Geometry: see drawing. Coordinates: mm, zero at the bounding-box minimum. A direction names the side the tool comes from. Coordinates: 2 decimals unless noted, no trailing zeros. Loops run counter-clockwise (first coordinate to the right, second up) from the corner with the lowest first, then second, coordinate; pieces in that order, holes last. Notation, with made-up numbers: (7.25, 13.25) - (57.25, 13.25) arc R17 ccw to (57.25, 35.25) - close; hole circle Ø8 at (-30.75, 9.25). An arc over 180 degrees is marked (long way). Answer in a Markdown table with one row per item.
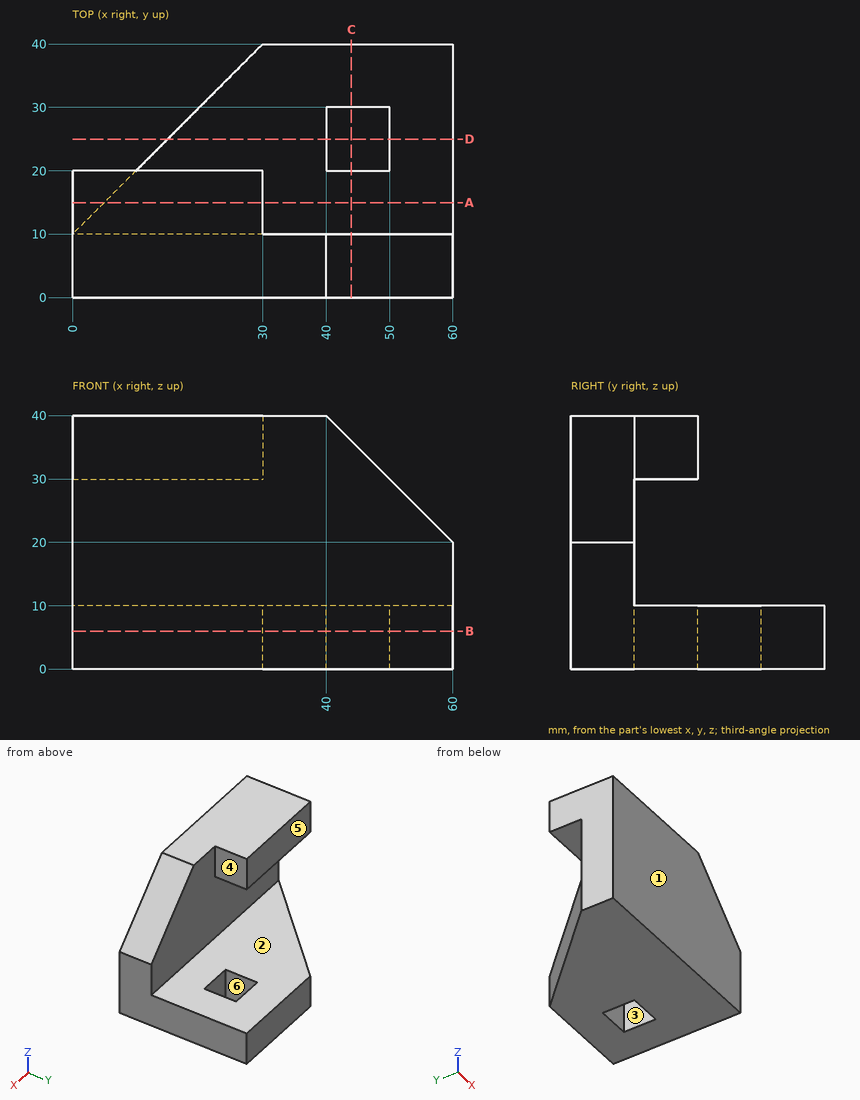
(1) Pull-direction query (Y, two-part tool) for the marked faces 4, 5 and 6; classes: pulls with the +Y half, pulls with the -Y half, needs draft (parallel to the pull), parting line crosses it, or undercut.
Verdict:
| item | result |
|---|---|
| face 4 | needs draft |
| face 5 | pulls with the +Y half |
| face 6 | undercut |
(2) Cut plane C-C on x = 44. Output: boundary loops of the cut face in (y, z), then the cut area to 3 significant figures.
Verdict:
| item | result |
|---|---|
| outline | (0, 0) - (20, 0) - (20, 10) - (10, 10) - (10, 36) - (0, 36) - close; (30, 0) - (40, 0) - (40, 10) - (30, 10) - close |
| area | 560 mm² |
(3) Ray query, probe 1 along Z at (x, y) = (19, 17); probe 2 along Y at (x, z) = (12, 11); probe 3 along Y at (x, z) = (40.5, 4.5). Return the intervals inside material, ascending.
Verdict:
| item | result |
|---|---|
| probe 1 | z = 0 to 10, 30 to 40 |
| probe 2 | y = 0 to 10 |
| probe 3 | y = 0 to 20, 30 to 40 |
(4) Cut plane D-D on y = 25. Output: boundary loops of the cut face in (x, z), then the cut area to 3 significant figures.
Verdict:
| item | result |
|---|---|
| outline | (15, 0) - (40, 0) - (40, 10) - (15, 10) - close; (50, 0) - (60, 0) - (60, 10) - (50, 10) - close |
| area | 350 mm² |
(5) Access query for the marked faces 1, 2 and 3. Directions: +Z, -Z, +X, -X, +Y, -Y. A direction counts if a zero-diameter tool reaches every point of the face in a straight line with its end or side. Return the directions, or none.
Verdict:
| item | result |
|---|---|
| face 1 | +Z, -Z, +X, -X, -Y |
| face 2 | +X, -X, +Y |
| face 3 | +Z, -Z |
(6) Cut plane A-A on y = 15. Output: boundary loops of the cut face in (x, z).
Verdict:
| item | result |
|---|---|
| outline | (0, 30) - (30, 30) - (30, 40) - (0, 40) - close; (5, 0) - (60, 0) - (60, 10) - (5, 10) - close |
(7) First-contact query: pin 1 Ø6 at (y, z) = (28.5, 15.5) entering from +X; pin 2 Ø5 at (x, z) = (13, 36) entering from +Y; pin 3 Ø8 at (y, z) = (22.5, 4) entering from -X; pin 4 Ø5 at (y, z) = (15.5, 37) entering from +X. Flat tips, straight axial feed; report the tip coordinate or a pass-through.
Verdict:
| item | result |
|---|---|
| pin 1 | passes through |
| pin 2 | stops at y = 20 |
| pin 3 | stops at x = 8.5 |
| pin 4 | stops at x = 30 |
(8) Cut plane B-B on z = 6. Output: boundary loops of the cut face in (x, y).
Verdict:
| item | result |
|---|---|
| outline | (0, 0) - (60, 0) - (60, 40) - (30, 40) - (0, 10) - close; hole (40, 20) - (50, 20) - (50, 30) - (40, 30) - close |
